Autodesk Inventor part; units mm, degrees
ref_plane "YZ Plane" through (0, 0, 0) normal (1, 0, 0) x (0, 1, 0)
ref_plane "XZ Plane" through (0, 0, 0) normal (0, 1, 0) x (-1, 0, 0)
ref_plane "XY Plane" through (0, 0, 0) normal (0, 0, 1) x (1, 0, 0)
sketch "Sketch1" plane through (0, 0, 0) normal (0, 0, 1) x (1, 0, 0)
  arc A0 (19.685, 0) -> (-19.685, 0) centre (0, 0) ccw
  arc A1 (28.6435, 9.652) -> (-30.226, 0) centre (0, 0) ccw
  line L0 (44.45, 0) -> (44.45, 9.652)
  line L1 (44.45, 9.652) -> (28.6435, 9.652)
  line L2 (-30.226, 0) -> (-19.685, 0)
  line L3 (19.685, 0) -> (44.45, 0)
  dimension "d0" = 39.37
  dimension "d1" = 60.452
  dimension "d2" = 44.45
  dimension "d15" = 9.652
extrude "Extrusion1" add sketch "Sketch1" against normal blind 12.7
fillet "Fillet1" radius 3.175 1 edges at (28.6435, 9.652, -6.35)
sketch "Sketch2" plane through (44.45, 9.652, 0) normal (0, 1, 0) x (1, 0, 0)
  line L0 (0, 0) -> (0, 12.7)
  line L1 (-13.6102, 12.7) -> (0, 12.7)
  point P0 (-44.45, 0)
  point P1 (-6.35, 6.35)
  dimension "d6" = 6.35
  dimension "d7" = 6.35
hole "Hole1" at (38.1, 9.652, -6.35) direction (0, -1, 0) diameter 6.858 end through all
properties part number "GE-13039" material "Polycarbonate, Clear"
The listing builds one solid part. Answer for the finished solid, in the listing's coordinates (mm). Coordinates: 2 decimals unless noted, no trailing zeros. Order: outer loops, then holes, each group sorted by start corner. A loop starts at its lowest first (then second) coordinate and runs counter-clockwise, first axis right, second up. Notation, with made-up numbers: M 76,70.25 L 88,70.25 A27 ccw 88,98.25 Z; hole C 56.5,79 d4. An arc over 180 degrees is marked long. Answer as a JSON object with one key per item and string values. Group by question number.
1. Section A-A on x = 38.1 is taken. Write down the section's boundary in (y, z), then the cut area to 3 significant figures.
2. Determine the mould class of faces 1 (the cylindrical face through (34.7, 4.8, -6.8)), 2 (the flat face through (36, 9.652, -3)), 3 (the flat face through (7, 19, 0)) for opening direction Z: released by +Z, released by -Z, zero draft, split by the parting line, or undercut.
3. Section D-D on y = 14.5 is taken. Write down the section's boundary in (x, z), then the cut area to 3 significant figures.
4. Flat-ended cylindrical pins translate along their axes: P1, Ø4, axis at x = 38.1, z = -6.35, coming from the -Y side; P2, Ø2, axis at x = 25, z = -7.5, coming from the +Y side; P3, Ø1, axis at x = 37, z = -10.5, coming from the +Y side; P4, Ø3, axis at x = 2, z = -5, coming from the -Y side. Find the tip coordinate at first contact, or state that the pin passes through.
5. Straight lines are drawn through the part: line 1 (Z direction, x = 38.1, y = 7); line 2 (X direction, y = 6.5, z = -6.35); line 3 (X direction, y = 4.5, z = -6.35). For each, find the intervals that lie inside material, in ascending order.
6. Section B-B on y = 7.5 is taken. Write down the section's boundary in (x, z), then the cut area to 3 significant figures.
7. Section C-C on z = -6.35 is taken. Write down the section's boundary in (x, y) (3 decimals), then the cut area to 3 significant figures.
Values follow:
{
 "1": {"outline": "M 0,-12.7 L 9.65,-12.7 L 9.65,-9.78 L 0,-9.78 Z; M 0,-2.92 L 9.65,-2.92 L 9.65,0 L 0,0 Z", "area": "56.4 mm2"},
 "2": {"face 1": "undercut", "face 2": "zero draft", "face 3": "released by +Z"},
 "3": {"outline": "M -26.52,-12.7 L -13.31,-12.7 L -13.31,0 L -26.52,0 Z; M 13.31,-12.7 L 26.52,-12.7 L 26.52,0 L 13.31,0 Z", "area": "335 mm2"},
 "4": {"P1": "through", "P2": "y = 18.37", "P3": "y = 9.65", "P4": "y = 19.37"},
 "5": {"line 1": "-12.7 to -9.78, -2.92 to 0", "line 2": "-29.52 to -18.58, 18.58 to 34.67, 41.53 to 44.45", "line 3": "-29.89 to -19.16, 19.16 to 34.67, 41.53 to 44.45"},
 "6": {"outline": "M -29.28,-12.7 L -18.2,-12.7 L -18.2,0 L -29.28,0 Z; M 18.2,-12.7 L 44.45,-12.7 L 44.45,0 L 18.2,0 Z; hole C 38.1,-6.35 d6.86", "area": "437 mm2"},
 "7": {"outline": "M -30.226,0 L -19.685,0 A19.685 cw 19.685,0 L 34.671,0 L 34.671,9.652 L 30.84,9.652 A3.175 cw 27.908,11.608 A30.226 ccw Z; M 41.529,0 L 44.45,0 L 44.45,9.652 L 41.529,9.652 Z", "area": "903 mm2"}
}
